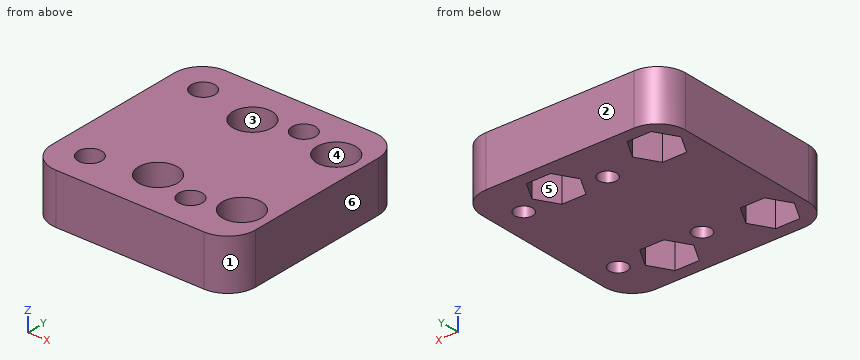
from build123d import *

# Parameters (mm, degrees)
SKETCH1_W           = 36.5
SKETCH1_H           = 36
SKETCH1_R           = 1.625
SKETCH1_R_2         = 2.125
BOSS_EXTRUDE1_DEPTH = 9
SKETCH2_R           = 3.5
CUT_EXTRUDE1_DEPTH  = 5
CUT_EXTRUDE2_DEPTH  = 5
FILLET2_R           = 5


with BuildPart() as part:
    # Sketch1 → Boss-Extrude1 (new body)
    with BuildSketch(Plane.XY):
        with Locations((1.75, 10)):
            Rectangle(SKETCH1_W, SKETCH1_H)
        with Locations((0, 20)):
            Circle(SKETCH1_R, mode=Mode.SUBTRACT)
        with Locations((15, 20)):
            Circle(SKETCH1_R, mode=Mode.SUBTRACT)
        with Locations((15, 0)):
            Circle(SKETCH1_R, mode=Mode.SUBTRACT)
        Circle(SKETCH1_R, mode=Mode.SUBTRACT)
        with Locations((-10.5, 22)):
            Circle(SKETCH1_R_2, mode=Mode.SUBTRACT)
        with Locations((7.5, 22)):
            Circle(SKETCH1_R_2, mode=Mode.SUBTRACT)
        with Locations((7.5, -2)):
            Circle(SKETCH1_R_2, mode=Mode.SUBTRACT)
        with Locations((-10.5, -2)):
            Circle(SKETCH1_R_2, mode=Mode.SUBTRACT)
    extrude(amount=BOSS_EXTRUDE1_DEPTH)

    # Sketch2 → Cut-Extrude1 (cut)
    with BuildSketch(Plane.XY.offset(9)):
        with Locations((0, 20)):
            Circle(SKETCH2_R)
        Circle(SKETCH2_R)
        with Locations((15, 0)):
            Circle(SKETCH2_R)
        with Locations((15, 20)):
            Circle(SKETCH2_R)
    extrude(amount=-CUT_EXTRUDE1_DEPTH, mode=Mode.SUBTRACT)

    # Sketch3 → Cut-Extrude2 (cut)
    with BuildSketch(Plane(origin=(0, 0, 0), x_dir=(-1, 0, 0), z_dir=(0, 0, -1))):
        Polygon((-5.334936491, 18.25), (-3.169872981, 22), (-5.334936491, 25.75), (-9.665063509, 25.75), (-11.830127019, 22), (-9.665063509, 18.25), align=None)
        Polygon((12.665063509, 18.25), (14.830127019, 22), (12.665063509, 25.75), (8.334936491, 25.75), (6.169872981, 22), (8.334936491, 18.25), align=None)
        Polygon((12.665063509, -5.75), (14.830127019, -2), (12.665063509, 1.75), (8.334936491, 1.75), (6.169872981, -2), (8.334936491, -5.75), align=None)
        Polygon((-9.665063509, -5.75), (-5.334936491, -5.75), (-3.169872981, -2), (-5.334936491, 1.75), (-9.665063509, 1.75), (-11.830127019, -2), align=None)
    extrude(amount=-CUT_EXTRUDE2_DEPTH, mode=Mode.SUBTRACT)

    # Fillet2
    fillet2_edges = [part.edges().sort_by_distance(p)[0] for p in [
        (-16.5, 28, 4.5),
        (20, 28, 4.5),
        (20, -8, 4.5),
        (-16.5, -8, 4.5),
    ]]
    fillet(fillet2_edges, radius=FILLET2_R)


solid = part.part
Verification items for the finished model (mm, model axes). Face numbers are marked on the shaded views. A direction names the side the tool comes from. Coordinates: 2 decimals unless noted, no trailing zeros. Write each loop counter-clockwise with the first axis right and the second up, starting at its lowest first coordinate (ties: lowest second). Pieces come first, ordered by that corner, then holes. Notation, with made-up numbers: M 19,2 L 51,2 A36 cw 51,41 Z; hole C 71,42.25 d2. An arc over 180 degrees is marked long. Use a Markdown table: item, result.
Q1. Set-up check for the marked faces 4, 5 and 6: record each of +Z, -Z, +X, -X, +Y, -Y from which the full face is reachable in a straight line by a thin tool's end or side.
Reply:
| item | result |
|---|---|
| face 4 | +Z |
| face 5 | -Z |
| face 6 | +Z, -Z, +X, +Y, -Y |
Q2. Sectioned sample at A-A, the plane x = -10.5. Record the boundary of the cut face in (y, z) (3 decimals), plus the area to 3 significant figures.
Reply:
| item | result |
|---|---|
| outline | M -8,0 L -5.75,0 L -5.75,5 L -4.125,5 L -4.125,9 L -8,9 Z; M 0.125,5 L 1.75,5 L 1.75,0 L 18.25,0 L 18.25,5 L 19.875,5 L 19.875,9 L 0.125,9 Z; M 24.125,5 L 25.75,5 L 25.75,0 L 28,0 L 28,9 L 24.125,9 Z |
| area | 215 mm² |
Q3. Sectioned sample at D-D, the plane y = 19. Record the boundary of the cut face in (x, z), plus the area to 3 significant figures.
Reply:
| item | result |
|---|---|
| outline | M -16.5,0 L -13.1,0 L -13.1,5 L -7.9,5 L -7.9,0 L -1.28,0 L -1.28,4 L -3.35,4 L -3.35,9 L -16.5,9 Z; M 1.28,0 L 4.9,0 L 4.9,5 L 10.1,5 L 10.1,0 L 13.72,0 L 13.72,4 L 11.65,4 L 11.65,9 L 3.35,9 L 3.35,4 L 1.28,4 Z; M 16.28,0 L 20,0 L 20,9 L 18.35,9 L 18.35,4 L 16.28,4 Z |
| area | 189 mm² |
Q4. Sectioned sample at C-C, the plane x = 0. Record the boundary of the cut face in (y, z) (3 decimals).
Reply:
| item | result |
|---|---|
| outline | M -8,0 L -1.625,0 L -1.625,4 L -3.5,4 L -3.5,9 L -8,9 Z; M 1.625,0 L 18.375,0 L 18.375,4 L 16.5,4 L 16.5,9 L 3.5,9 L 3.5,4 L 1.625,4 Z; M 21.625,0 L 28,0 L 28,9 L 23.5,9 L 23.5,4 L 21.625,4 Z |
Q5. Go/stop test with flat-tipped pins: P1, Ø4, axis at x = 7.5, y = -2, coming from the -Z side; P2, Ø5.5, axis at x = 15, y = 20, coming from the +Z side; P3, Ø2, axis at x = -12, y = 20.5, coming from the -Z side. Record where each tip stops, or that it passes through.
Reply:
| item | result |
|---|---|
| P1 | passes through |
| P2 | stops at z = 4 |
| P3 | stops at z = 5 |
Q6. Draft check along Y on the marked faces 1, 2 and 3. Enter one of: +Y half, -Y half, draft (parallel to the pull), parting line (faces both ways), or undercut.
Reply:
| item | result |
|---|---|
| face 1 | -Y half |
| face 2 | +Y half |
| face 3 | undercut |
Q7. Sectioned sample at B-B, the plane z = 7.25. Count the separate pieces of the cut face and the enclosed holes in it, plus the area to 3 significant figures.
Reply:
| item | result |
|---|---|
| separate pieces | 1 |
| enclosed holes | 8 |
| area | 1,080 mm² |
Q8. Thickness scan on line 1 (Y direction, x = 15, z = 6.6); line 2 (Y direction, x = 6.5, z = 2.25); line 3 (X direction, y = 22, z = 2.25). Record the ranges inside material, lowest first.
Reply:
| item | result |
|---|---|
| line 1 | y = -8 to -3.5, 3.5 to 16.5, 23.5 to 28 |
| line 2 | y = -8 to -5.75, 1.75 to 18.25, 25.75 to 28 |
| line 3 | x = -16.5 to -14.83, -6.17 to 3.17, 11.83 to 20 |
